The model under review builds one solid part; all positions refer to its coordinate system, in mm. Face numbers are marked on the shaded views. A direction names the side the tool comes from. Give positions to 0.01 mm unless a question says otherwise; leave off trailing zeros. Loops run counter-clockwise (first coordinate to the right, second up) from the corner with the lowest first, then second, coordinate; pieces in that order, holes last. Notation, with made-up numbers: M -28,47.5 L 17,47.5 A19 ccw 17,56.5 Z; hole C -8.75,57.5 d4. An arc over 180 degrees is marked long. One line per item, written item: value. Start each with the question number.
Q1. For the marked faces 1 and 2, list the 3-axis set-ups (+Z, -Z, +X, -X, +Y, -Y) from which the entire face can be reached by the end or side of a thin tool; tool diameter is ignored.
Q2. We need section C-C on y = 1.25. Write out the cut boundary in (x, z), plus the area to 3 significant figures.
Q3. For pin 1 (10 mm diameter, centred on x = -1, z = 7.5, fed in from -Y); pin 2 (1 mm diameter, centred on y = 1, z = 10, fed in from -X); pin 3 (4 mm diameter, centred on y = -1.5, z = -19, fed in from +X), all flat-tipped, find the tip position at first contact; note any pin that passes through.
Q4. We need section D-D on x = 0. Write out the cut boundary in (y, z) (3 decimals), plus the area to 3 significant figures.
Q5. Mouldability with a two-part tool opening along Z and no side actions: class the marked faces 3 and 4 as released by +Z, released by -Z, zero draft, split by the parting line, or undercut.
Q6. We need section A-A on x = 15. Write out the cut boundary in (y, z), plus the area to 3 significant figures.
Q7. We need section B-B on z = 18.5. Write out the cut boundary in (x, y), plus the area to 3 significant figures.
Q8. To check wall thickness, follow line 1 along Z through (x, y) = (0, -3.35) (3 decimals); line 2 along Z through (x, y) = (0, -1.2); line 3 along Z through (x, y) = (3, -4). State the ranges of each line that lie inside material, in increasing order. Write a range as from..to.
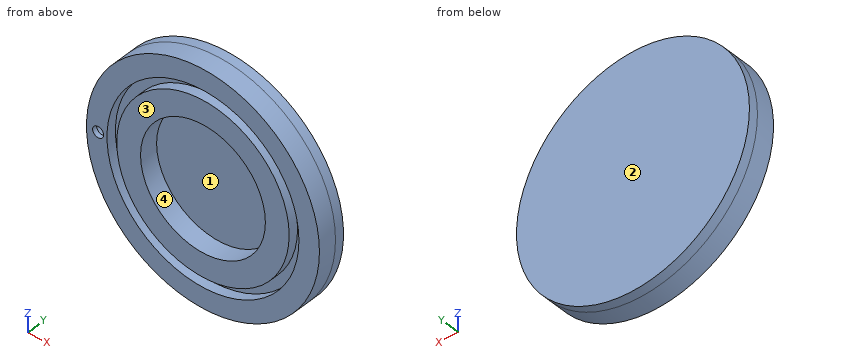
Autodesk Inventor part; units mm, degrees
ref_plane "YZ Plane" through (0, 0, 0) normal (1, 0, 0) x (0, 1, 0)
ref_plane "XZ Plane" through (0, 0, 0) normal (0, 1, 0) x (-1, 0, 0)
ref_plane "XY Plane" through (0, 0, 0) normal (0, 0, 1) x (1, 0, 0)
sketch "Sketch1" plane through (0, 0, 0) normal (0, 1, 0) x (-1, 0, 0)
  circle A0 centre (0, 0) radius 31.75
  dimension "d0" = 63.5
extrude "Extrusion1" add sketch "Sketch1" along normal blind 2.54
sketch "Sketch2" plane through (0, 0, 0) normal (0, -1, 0) x (1, 0, 0)
  circle A0 centre (0, 0) radius 31.75
  circle A1 centre (0, 0) radius 17.018
  circle A2 centre (0, 0) radius 31.75
  dimension "d4" = 34.036
extrude "Extrusion2" add sketch "Sketch2" along normal blind 5.08
sketch "Sketch3" plane through (0, -5.08, 0) normal (0, -1, 0) x (1, 0, 0)
  circle A0 centre (0, 0) radius 23.495
  circle A1 centre (0, 0) radius 17.018
  circle A2 centre (0, 0) radius 26.162
  dimension "d7" = 46.99
  dimension "d8" = 52.324
extrude "Extrusion3" cut sketch "Sketch3" against normal blind 2.667 contours A2
sketch "Sketch5" plane through (0, -5.08, 0) normal (0, -1, 0) x (1, 0, 0)
  point P0 (0, 0)
  point P1 (-28.575, 0)
  dimension "d18" = 28.575
hole "Hole1" at (-28.575, -5.08, 0) direction (0, 1, 0) diameter 3 depth 1.27 tip angle 118
properties part number "LED housing the one we're using"
Solved:
1. face 1: -Y
1. face 2: +Z, -Z, +X, -X, +Y
2. outline: C 0,0 d63.5
2. area: 3,170 mm2
3. pin 1: y = 0
3. pin 2: x = -30.3
3. pin 3: x = 26.82
4. outline: M -5.08,-31.75 L 2.54,-31.75 L 2.54,31.75 L -5.08,31.75 L -5.08,26.162 L -2.413,26.162 L -2.413,23.495 L -5.08,23.495 L -5.08,17.018 L 0,17.018 L 0,-17.018 L -5.08,-17.018 L -5.08,-23.495 L -2.413,-23.495 L -2.413,-26.162 L -5.08,-26.162 Z
4. area: 297 mm2
5. face 3: zero draft
5. face 4: undercut
6. outline: M -5.08,-27.98 L 2.54,-27.98 L 2.54,27.98 L -5.08,27.98 L -5.08,21.43 L -2.41,21.43 L -2.41,18.08 L -5.08,18.08 L -5.08,8.04 L 0,8.04 L 0,-8.04 L -5.08,-8.04 L -5.08,-18.08 L -2.41,-18.08 L -2.41,-21.43 L -5.08,-21.43 Z
6. area: 327 mm2
7. outline: M -25.8,-5.08 L -18.5,-5.08 L -18.5,-2.41 L -14.48,-2.41 L -14.48,-5.08 L 14.48,-5.08 L 14.48,-2.41 L 18.5,-2.41 L 18.5,-5.08 L 25.8,-5.08 L 25.8,2.54 L -25.8,2.54 Z
7. area: 372 mm2
8. line 1: -31.75..-26.162, -23.495..-17.018, 17.018..23.495, 26.162..31.75
8. line 2: -31.75..-17.02, 17.02..31.75
8. line 3: -31.61..-25.99, -23.3..-16.75, 16.75..23.3, 25.99..31.61
